Build history of the part. All positions in model axes, mm. A direction names the side the tool comes from. Give positions to 0.01 mm unless a question says otherwise; leave off trailing zeros. Order: outer loops, then holes, each group sorted by start corner. A loop starts at its lowest first (then second) coordinate and runs counter-clockwise, first axis right, second up. Notation, with made-up numbers: M 80.25,-32.75 L 126.25,-32.75 A19 cw 126.25,-19.75 Z; hole C -5.75,68 d2. An arc over 180 degrees is marked long. Answer as CSV lines item,"result".
from build123d import *

# Parameters (mm, degrees)
SKETCH1_W           = 35
SKETCH1_H           = 9
BOSS_EXTRUDE1_DEPTH = 3
BOSS_EXTRUDE2_DEPTH = 12
CHAMFER1_SIZE       = 1


with BuildPart() as part:
    # Sketch1 → Boss-Extrude1 (new body)
    with BuildSketch(Plane(origin=(0, 0, 0), x_dir=(1, 0, 0), z_dir=(0, 1, 0))):
        with Locations((17.5, 4.5)):
            Rectangle(SKETCH1_W, SKETCH1_H)
    extrude(amount=BOSS_EXTRUDE1_DEPTH)

    # Sketch2 → Boss-Extrude2 (add)
    with BuildSketch(Plane(origin=(0, 3, 0), x_dir=(1, 0, 0), z_dir=(0, 1, 0))):
        Polygon((0, 9), (35, 9), (35, 6), (35, 5.5), (32, 5.5), (32, 6), (3, 6), (3, 5.5), (0, 5.5), (0, 6.813124062), align=None)
        Polygon((0, 0), (35, 0), (35, 3), (35, 3.5), (32, 3.5), (32, 3), (3, 3), (3, 3.5), (0, 3.5), (0, 2.186875938), align=None)
    extrude(amount=BOSS_EXTRUDE2_DEPTH)

    # Chamfer1
    chamfer1_edges = [part.edges().sort_by_distance(p)[0] for p in [
        (0, 15, -7.25),
        (1.5, 15, -5.5),
        (3, 15, -5.75),
        (17.5, 15, -6),
        (32, 15, -5.75),
        (33.5, 15, -5.5),
        (35, 15, -7.25),
        (17.5, 15, -9),
        (0, 15, -1.75),
        (17.5, 15, 0),
        (35, 15, -1.75),
        (33.5, 15, -3.5),
        (32, 15, -3.25),
        (17.5, 15, -3),
        (3, 15, -3.25),
        (1.5, 15, -3.5),
    ]]
    chamfer(chamfer1_edges, length=CHAMFER1_SIZE)


solid = part.part
Item 1: Band-saw the part on C-C (z = -0.5). Give the cut face in (x, y).
Geometry says:
outline,"M 0,0 L 35,0 L 35,14 L 34.5,14.5 L 0.5,14.5 L 0,14 Z"
Item 2: Band-saw the part on D-D (x = 15). Give the cut face in (y, z).
Geometry says:
outline,"M 0,-9 L 14,-9 L 15,-8 L 15,-7 L 14,-6 L 3,-6 L 3,-3 L 14,-3 L 15,-2 L 15,-1 L 14,0 L 0,0 Z"
Item 3: Pull direction Z, two halves, no side cores. Call faces 1 (the flat face through (17, 7, 0)), 2 (the flat face through (33.5, 14.4, -5.9)), 3 (the flat face through (32.5, 14.5, -2.8)), 4 (the flat face through (0.4, 14.4, -7.3)): released by +Z, released by -Z, zero draft, split by the parting line, or undercut.
Geometry says:
face 1,"released by +Z"
face 2,"undercut"
face 3,"undercut"
face 4,"zero draft"
Item 4: 3-axis set-ups, long thin cutter, end or side, ignore diameter. For faces 5 (the flat face through (32.5, 14.5, -6.2)), 6 (the flat face through (34.6, 14.4, -7.2)), 7 (the flat face through (2, 8, -5.5)): which of +Z, -Z, +X, -X, +Y, -Y reach the whole face in a straight line?
Geometry says:
face 5,"+Y"
face 6,"+Z, -Z, +X, +Y"
face 7,"+X, -X, +Y"
Item 5: Band-saw the part on A-A (y = 6.5). Give the cut face in (x, z), and give its area (3 significant figures).
Geometry says:
outline,"M 0,-9 L 35,-9 L 35,-5.5 L 32,-5.5 L 32,-6 L 3,-6 L 3,-5.5 L 0,-5.5 Z; M 0,-3.5 L 3,-3.5 L 3,-3 L 32,-3 L 32,-3.5 L 35,-3.5 L 35,0 L 0,0 Z"
area,"216 mm2"
Item 6: Drop flat-ended pins along their axis: pin 1 (1.5 mm diameter, centred on x = 12.5, z = -4.5, fed in from +Y); pin 2 (6 mm diameter, centred on x = 11.5, y = 4.5, fed in from +Z). Give the stop position or say it passes through.
Geometry says:
pin 1,"stops at y = 3"
pin 2,"stops at z = 0"
Item 7: Probe line 1 along Z through (x, y) = (5.5, 12); line 2 along Y through (x, z) = (18, -5.75); line 3 along Z through (x, y) = (33, 13.75). List the from-to ranges inside material, lowest first. Write a range as from..to.
Geometry says:
line 1,"z = -9..-6, -3..0"
line 2,"y = 0..3"
line 3,"z = -9..-5.5, -3.5..0"
Item 8: Band-saw the part on B-B (x = 2.5). Give the cut face in (y, z).
Geometry says:
outline,"M 0,-9 L 14,-9 L 15,-8 L 15,-7 L 14.5,-6.5 L 14.5,-6 L 14,-5.5 L 3,-5.5 L 3,-3.5 L 14,-3.5 L 14.5,-3 L 14.5,-2.5 L 15,-2 L 15,-1 L 14,0 L 0,0 Z"
